Work out the finished part from the listing and answer in its coordinate system (mm). Coordinates: 2 decimals unless noted, no trailing zeros. Order: outer loops, then holes, each group sorted by start corner. A loop starts at its lowest first (then second) coordinate and runs counter-clockwise, first axis right, second up.
1. The part is cut by section B-B, the plane x = -224. Give the vertices of the cut face in (y, z), then the cut area to 3 significant figures.
2. The part is cut by section A-A, the plane y = 13. Give the vertices of the cut face in (x, z), then the cut area to 3 significant figures.
3. The part is cut by section D-D, the plane x = -166. Give the vertices of the cut face in (y, z), then the cut area to 3 significant figures.
4. The part is cut by section C-C, the plane z = -191.4. Count the separate pieces of the cut face and the enclosed holes in it, then the cut area to 3 significant figures.
5. Find the intervals of material crossed by probe 1 along Y at (x, z) = (-215, -193.9); probe 2 along X at (y, z) = (47.5, -190); probe 3 along X at (y, z) = (51.5, -190.5), in increasing order.
```python
from build123d import *

# Parameters (mm, degrees)
SKETCH3_R             = 6.350000004
SKETCH3_R_2           = 3.25
SKETCH3_R_3           = 20.005589459
BOSS_EXTRUDE1_DEPTH   = 4.7625
FILLET1_R             = 3.175
FILLET2_R             = 5.08
M5_TAPPED_HOLE1_D     = 4.2
M5_TAPPED_HOLE1_DEPTH = 14
M5_TAPPED_HOLE1_TIP   = 1.2618073


with BuildPart() as part:
    # Sketch3 → Boss-Extrude1 (new body)
    with BuildSketch(Plane.XY.offset(-194.177612449)):
        Polygon((-209.572241428, 79.105126535), (-129.572241428, 70.355126535), (-129.572241428, 30.355126535), (-169.572241428, -9.644873465), (-209.572241428, -9.644873465), (-266.721169677, 21.605126535), (-266.721169677, 78.755126535), align=None)
        with Locations(Location((-189.572241428, 10.355126535, 0), (0, 0, 180))):
            Circle(SKETCH3_R, mode=Mode.SUBTRACT)
        with Locations(Location((-182.572241428, 50.355126535, 0), (0, 0, 180))):
            Circle(SKETCH3_R_2, mode=Mode.SUBTRACT)
        with Locations(Location((-144.572241428, 50.355126535, 0), (0, 0, 180))):
            Circle(SKETCH3_R_2, mode=Mode.SUBTRACT)
        with Locations(Location((-238.146169677, 50.180126535, 0), (0, 0, 180))):
            Circle(SKETCH3_R_3, mode=Mode.SUBTRACT)
    extrude(amount=BOSS_EXTRUDE1_DEPTH)

    # Fillet1
    fillet1_edges = [part.edges().sort_by_distance(p)[0] for p in [
        (-209.572241428, -9.644873465, -191.796362449),
        (-169.572241428, -9.644873465, -191.796362449),
        (-129.572241428, 30.355126535, -191.796362449),
        (-129.572241428, 70.355126535, -191.796362449),
    ]]
    fillet(fillet1_edges, radius=FILLET1_R)

    # Fillet2
    fillet2_edges = [part.edges().sort_by_distance(p)[0] for p in [
        (-266.721169677, 78.755126535, -191.796362449),
        (-266.721169677, 21.605126535, -191.796362449),
        (-209.572241428, 79.105126535, -191.796362449),
    ]]
    fillet(fillet2_edges, radius=FILLET2_R)

    # M5 Tapped Hole1
    with Locations(Plane.XY.offset(-189.415112449)):
        with Locations((-214.522241428, 74.124718176), (-261.771169677, 73.835349234), (-214.522241428, 26.555126535), (-261.771169677, 26.555126535)):
            Hole(M5_TAPPED_HOLE1_D / 2, depth=M5_TAPPED_HOLE1_DEPTH)
            with Locations((0, 0, -(M5_TAPPED_HOLE1_DEPTH + M5_TAPPED_HOLE1_TIP / 2))):  # 118° drill point
                Cone(0, M5_TAPPED_HOLE1_D / 2, M5_TAPPED_HOLE1_TIP, mode=Mode.SUBTRACT)


solid = part.part
```
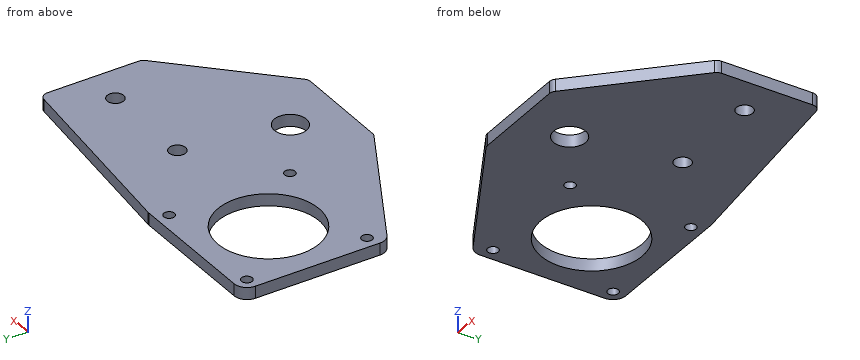
Geometry says:
1. outline: (-1.76, -194.18) - (36.03, -194.18) - (36.03, -189.42) - (-1.76, -189.42) - close; (64.33, -194.18) - (79.02, -194.18) - (79.02, -189.42) - (64.33, -189.42) - close
1. area: 250 mm2
2. outline: (-250.98, -194.18) - (-195.35, -194.18) - (-195.35, -189.42) - (-250.98, -189.42) - close; (-183.8, -194.18) - (-146.93, -194.18) - (-146.93, -189.42) - (-183.8, -189.42) - close
2. area: 441 mm2
3. outline: (-6.07, -194.18) - (74.34, -194.18) - (74.34, -189.42) - (-6.07, -189.42) - close
3. area: 383 mm2
4. separate pieces: 1
4. enclosed holes: 8
4. area: 8,600 mm2
5. probe 1: y = -6.68 to 24.51, 28.6 to 72.08, 76.17 to 79.07
5. probe 2: x = -266.72 to -257.97, -218.32 to -184.12, -181.02 to -146.12, -143.02 to -129.57
5. probe 3: x = -266.72 to -258.11, -218.18 to -185.61, -179.53 to -147.61, -141.53 to -129.57
